Check sheet for the modelled part. Datum: model origin and axes. Units: mm. A direction names the side the tool comes from. Give positions to 0.01 mm unless a question says otherwise; leave off trailing zeros. Order: outer loops, then holes, each group sorted by start corner. A loop starts at its lowest first (then second) coordinate and runs counter-clockwise, first axis right, second up. Notation, with made-up numbers: (83.5, 66.25) -> (104.5, 66.25) arc R14 ccw to (104.5, 91.25) -> close; hole circle Ø10 at (42, 15). An arc over 180 degrees is marked (long way). Answer in a Markdown table with one row per item. Add a question column.
(1) Thickness scan on L1, parallel to Y at x = -17, z = 15; L2, parallel to Z at x = -15, y = 26.9; L3, parallel to Z at x = 12, y = -4.5. Record the ranges inside material, lowest first. Write a range as [from, to].
(2) Go/stop test with flat-tipped pins: pin 1 (12 mm diameter, centred on x = 32, y = 9.5, fed in from +Z); pin 2 (10 mm diameter, centred on x = 3, z = 12.5, fed in from +Y); pin 3 (6 mm diameter, centred on x = 29, z = 12.5, fed in from +Y). Record where each tip stops, or that it passes through.
(3) Set-up check for faces 1 (the face through (22.59, 10.16, 5.29)), 2 (the face through (-12.56, -0.54, 27.6)), 3 (the face through (-13.74, 9.65, 23.28)): record each of +Z, -Z, +X, -X, +Y, -Y from which the full face is reachable in a straight line by a thin tool's end or side.
(4) Cross-section at A-A (x = -14). State how many separate pieces and enclosed holes the cut face has, then the cut area to 3 significant figures.
(5) Cross-section at C-C (x = 5.5). Record the cut outline in (y, z), then the cut area to 3 significant figures.
(6) Release check for a two-part mould opening along Z. For faces 4 (the face through (-26.505, -5, 27)), 5 (the face through (-12.56, 19.14, 19.9)), 6 (the face through (-10.996, 10.42, 5.42)), 7 (the face through (-29.55, 29.48, -6.55)) record: released by +Z, released by -Z, zero draft, split by the parting line, or undercut.
```python
from build123d import *

# Parameters (mm, degrees)
SKETCH4_R          = 2.5
CUT_EXTRUDE2_DEPTH = 100
CIRPATTERN2_COUNT  = 8


with BuildPart() as part:
    # Sketch1 → Revolve1 (revolve)
    with BuildSketch(Plane.XY, mode=Mode.PRIVATE) as revolve1_sk:
        with BuildLine():
            Line((1.039558454, 4.829261996), (46.348618443, 14.46))
            Line((46.348618443, 14.46), (46.348618443, 16.50468119))
            Line((46.348618443, 16.50468119), (7.917033014, 8.335795532))
            ThreePointArc((7.917033014, 8.335795532), (1.551763443, 8.363569436), (-4.228867695, 11.028476892))
            Line((-4.228867695, 11.028476892), (-18.261374171, 21.60272898))
            ThreePointArc((-18.261374171, 21.60272898), (-18.954391435, 23.834609313), (-17.057744125, 25.2))
            Line((-17.057744125, 25.2), (-10.504922768, 25.2))
            Line((-10.504922768, 25.2), (-10.504922768, 30.2))
            Line((-10.504922768, 30.2), (-22.504922768, 30.2))
            Line((-22.504922768, 30.2), (-22.504922768, 27.2))
            Line((-22.504922768, 27.2), (-26.504922768, 27.2))
            Line((-26.504922768, 27.2), (-26.504922768, 30.2))
            Line((-26.504922768, 30.2), (-32.504922768, 30.2))
            Line((-32.504922768, 30.2), (-32.504922768, 27.95353791))
            Line((-32.504922768, 27.95353791), (-3.009075116, 5.72682245))
            ThreePointArc((-3.009075116, 5.72682245), (-1.08219807, 4.838519964), (1.039558454, 4.829261996))
        make_face()
    revolve(revolve1_sk.sketch.rotate(Axis((-34.362308285, 0, 0), (1, 0, 0)), 90), axis=Axis((-34.362308285, 0, 0), (1, 0, 0)))

    # Sketch4 → Cut-Extrude2 (cut)
    with BuildSketch(Plane(origin=(0, 22, 0), x_dir=(-1, 0, 0), z_dir=(0, 1, 0))):
        with Locations(Location((15, 0, 0), (0, 0, 270))):
            Circle(SKETCH4_R)
    cut_extrude2 = extrude(amount=CUT_EXTRUDE2_DEPTH, mode=Mode.SUBTRACT)

    # CirPattern2: Cut-Extrude2 ×8 about axis
    cirpattern2_axis = Axis((-42.896286604, 0, 0), (1, 0, 0))
    for i in range(1, CIRPATTERN2_COUNT):
        add(cut_extrude2.rotate(cirpattern2_axis, i * 360 / CIRPATTERN2_COUNT), mode=Mode.SUBTRACT)


solid = part.part
```
Answer below:
| question | item | result |
|---|---|---|
| 1 | L1 | y = [-26.21, -20.25], [-14.2, -6.3], [6.3, 14.2], [20.25, 26.21] |
| 1 | L2 | z = [-13.73, -2.5], [2.5, 13.73] |
| 1 | L3 | z = [-8.03, -5.57], [5.57, 8.03] |
| 2 | pin 1 | stops at z = 13.43 |
| 2 | pin 2 | stops at y = 3.26 |
| 2 | pin 3 | stops at y = 8.74 |
| 3 | face 1 | none |
| 3 | face 2 | +Z |
| 3 | face 3 | +X |
| 4 | separate pieces | 9 |
| 4 | enclosed holes | 1 |
| 4 | area | 1,130 mm² |
| 5 | outline | circle Ø16.05 at (0, 0); hole circle Ø11.55 at (0, 0) |
| 5 | area | 97.4 mm² |
| 6 | face 4 | zero draft |
| 6 | face 5 | undercut |
| 6 | face 6 | undercut |
| 6 | face 7 | split by the parting line |
